from build123d import *

# Parameters (mm, degrees)
F0_R     = 10
F0_R_2   = 2.5
F0_R_3   = 0.75
F1_DEPTH = 10
F2_DEPTH = 8
F3_DEPTH = 10.5
F5_R     = 0.2


# Not quite as in the source:
# - a fillet or chamfer that OpenCascade refuses, or shapes differently, is made with other operations: its cross-section is extruded or revolved along the edge and cut away or added


with BuildPart() as f1:
    # F0 (on Top) → F1 (new body)
    with BuildSketch(Plane.XY):
        Circle(F0_R)
        Circle(F0_R_2, mode=Mode.SUBTRACT)
        with Locations((0, 8.75)):
            Circle(F0_R_3, mode=Mode.SUBTRACT)
        with Locations((0, 8.75)):
            Circle(F0_R_3)
        Circle(F0_R_2)
    extrude(amount=F1_DEPTH)

    # F0 (on Top) → F2 (cut)
    with BuildSketch(Plane.XY):
        Circle(F0_R_2)
    extrude(amount=F2_DEPTH, mode=Mode.SUBTRACT)

    # F0 (on Top) → F3 (join)
    with BuildSketch(Plane.XY):
        with Locations((0, 8.75)):
            Circle(F0_R_3)
    extrude(amount=F3_DEPTH)

    # F4: fillet of radius 0.798 on 1 edges, made by hand

    # F4_s1 → F4_t2 (revolve, cut)
    with BuildSketch(Plane.XZ.offset(-8.75)):
        with BuildLine():
            ThreePointArc((0.75, 10), (0.4563840077, 10.3632896491), (0.0097297791, 10.5))
            Line((0.0097297791, 10.5), (0.75, 10.5))
            Line((0.75, 10.5), (0.75, 10))
        make_face()
    revolve(axis=Axis((0, 8.75, 10.5), (0, 0, 1)), mode=Mode.SUBTRACT)

    # F5
    f5_edges = [f1.edges().sort_by_distance(p)[0] for p in [
        (-0.75, 8.75, 10),
    ]]
    fillet(f5_edges, radius=F5_R)


solid = f1.part
Geometry: final body of the model. Coordinates: model frame, mm. Give positions to 0.01 mm unless a question says otherwise; leave off trailing zeros. Write each loop counter-clockwise with the first axis right and the second up, starting at its lowest first coordinate (ties: lowest second). Pieces come first, ordered by that corner, then holes. Notation, with made-up numbers: (69, -23.5) - (94, -23.5) arc R34 ccw to (94, 10.5) - close; hole circle Ø6 at (60, 39). An arc over 180 degrees is marked (long way). Return JSON: item names as keys, results as strings. Group by question number.
1) Mould query, pull axis X, two halves, no side actions, for faces 1 (the flat face through (0, 0, 8)), 2 (the cylindrical face through (-0.54, -2.44, 3.94)), 3 (the cylindrical face through (-2.17, -9.76, 4.93)), 4 (the flat face through (2, -2, 0)). Classes: released by +X, released by -X, zero draft, split by the parting line, or undercut.
2) Section D-D on x = -2.75. Return the cut outline in (y, z), plus the area to 3 significant figures.
3) First-contact query: P1, Ø5, axis at x = 3.5, y = -4.5, coming from the +Z side; P2, Ø3, axis at x = 4, z = 6, coming from the +Y side; P3, Ø4, axis at x = -2.5, z = 8.5, coming from the +Y side. Flat tips, straight axial feed; report the tip coordinate or a pass-through.
4) Section B-B on z = 2.25. Return the cut outline in (x, y).
5) Section C-C on x = 8. Return the cut outline in (y, z), plus the area to 3 significant figures.
6) Section A-A on y = 0. Return the cut outline in (x, z).
7) Line query: line 1 (Y direction, x = 0, z = 6.75); line 2 (Z direction, x = 9, y = 3.5); line 3 (X direction, y = 1.75, z = 4.75). Output: solid intervals per line, ascending.
Filled in:
{
 "1": {"face 1": "undercut", "face 2": "undercut", "face 3": "split by the parting line", "face 4": "zero draft"},
 "2": {"outline": "(-9.61, 0) - (9.61, 0) - (9.61, 10) - (-9.61, 10) - close", "area": "192 mm^2"},
 "3": {"P1": "stops at z = 10", "P2": "stops at y = 9.68", "P3": "stops at y = 9.99"},
 "4": {"outline": "circle Ø20 at (0, 0); hole circle Ø5 at (0, 0)"},
 "5": {"outline": "(-6, 0) - (6, 0) - (6, 10) - (-6, 10) - close", "area": "120 mm^2"},
 "6": {"outline": "(-10, 0) - (-2.5, 0) - (-2.5, 8) - (2.5, 8) - (2.5, 0) - (10, 0) - (10, 10) - (-10, 10) - close"},
 "7": {"line 1": "y = -10 to -2.5, 2.5 to 10", "line 2": "z = 0 to 10", "line 3": "x = -9.85 to -1.79, 1.79 to 9.85"}
}
